Autodesk Fusion 360 part; units mm, degrees
sketch "Sketch1" plane through (0, 0, 0) normal (0, 0, 1) x (1, 0, 0)
  line L0 (-28, 37) -> (62, 37)
  line L1 (62, 37) -> (62, 18)
  line L2 (62, 18) -> (-28, 18)
  line L3 (-28, 18) -> (-28, 37)
  dimension "d1" = 90
  dimension "d2" = 19
extrude "Extrude1" add sketch "Sketch1" along normal blind 6
sketch "Sketch2" plane through (0, 0, 6) normal (0, 0, 1) x (-1, 0, 0)
  line L0 (28, -37) -> (28, -18)
  line L1 (28, -18) -> (-62, -18)
  line L2 (-62, -18) -> (-62, -37)
  line L3 (-62, -37) -> (28, -37)
ref_plane "WorkPlane1" through (17, 27.5, 6) normal (0, 0, 1) x (-1, 0, 0)
sketch "Sketch3" plane through (0, 0, 6) normal (0, 0, 1) x (1, 0, 0)
  line L0 (17, 37) -> (17, 18)
  circle A0 centre (-8, 27.5) radius 8.9
  circle A1 centre (42, 27.5) radius 8.9
  circle A2 centre (-8, 27.5) radius 3.65
  circle A3 centre (42, 27.5) radius 3.65
  dimension "d13" = 17.8
  dimension "d14" = 17.8
  dimension "d15" = 7.3
  dimension "d16" = 7.3
extrude "Extrude2" cut sketch "Sketch3" against normal blind 7 contours A2 | A3
extrude "Extrude3" cut sketch "Sketch3" against normal blind 3
sketch "Sketch4" plane through (0, 0, 0) normal (0, 0, 1) x (1, 0, 0)
  line L0 (-21, 37) -> (55, 37)
  line L1 (55, 37) -> (55, 39)
  line L2 (55, 39) -> (-21, 39)
  line L3 (-21, 39) -> (-21, 37)
  dimension "d21" = 76
  dimension "d22" = 2
sketch "Sketch7" plane through (0, 0, 6) normal (0, 0, 1) x (-1, 0, 0)
  circle A0 centre (-42, -27.5) radius 8.9
  circle A1 centre (8, -27.5) radius 8.9
  line L0 (28, -18) -> (-62, -18)
  line L1 (-62, -18) -> (-62, -37)
  line L2 (-62, -37) -> (28, -37)
  line L3 (28, -37) -> (28, -18)
  line L4 (28, -37) -> (-62, -37)
  line L5 (-62, -37) -> (-62, -73)
  line L6 (-62, -73) -> (28, -73)
  line L7 (28, -73) -> (28, -37)
  dimension "d37" = 90
  dimension "d38" = 36
extrude "Extrude7" add sketch "Sketch7" against normal blind 6 contours L2 L4 L5 L6 L7
sketch "Sketch8" plane through (0, 0, 6) normal (0, 0, 1) x (-1, 0, 0)
  circle A0 centre (-42, -27.5) radius 8.9
  circle A1 centre (8, -27.5) radius 8.9
  line L0 (28, -18) -> (-62, -18)
  line L1 (-62, -18) -> (-62, -73)
  line L2 (-62, -73) -> (28, -73)
  line L3 (28, -73) -> (28, -18)
  line L4 (-62, -18) -> (28, -18)
  line L5 (28, -18) -> (28, 18)
  line L6 (28, 18) -> (-62, 18)
  line L7 (-62, 18) -> (-62, -18)
  dimension "d41" = 90
  dimension "d42" = 36
extrude "Extrude8" add sketch "Sketch8" against normal blind 6 contours L0 L4 L5 L6 L7
ref_plane "WorkPlane3" through (17, 27.5, 6) normal (0, 0, 1) x (1, 0, 0)
sketch "Sketch9" plane through (0, 0, 6) normal (0, 0, 1) x (1, 0, 0)
  line L0 (62, -18) -> (-28, -18)
  line L1 (-28, -18) -> (-28, -14)
  line L2 (-28, -14) -> (62, -14)
  line L3 (62, -14) -> (62, -18)
  line L4 (62, 73) -> (-28, 73)
  line L5 (-28, 73) -> (-28, 69)
  line L6 (-28, 69) -> (62, 69)
  line L7 (62, 69) -> (62, 73)
  line L8 (62, -14) -> (62, -14)
  line L9 (62, 69) -> (62, 69)
  line L10 (62, -14) -> (58, -14)
  line L11 (58, -14) -> (58, 69)
  line L12 (58, 69) -> (62, 69)
  line L13 (62, 69) -> (62, -14)
  dimension "d46" = 90
  dimension "d47" = 4
  dimension "d48" = 90
  dimension "d49" = 4
  dimension "d50" = 83
extrude "Extrude9" add sketch "Sketch9" along normal blind 27
ref_plane "WorkPlane4" through (17, 27.5, 33) normal (0, 0, 1) x (1, 0, 0)
sketch "Sketch10" plane through (0, 0, 33) normal (0, 0, 1) x (1, 0, 0)
  line L0 (62, -18) -> (22, -18)
  line L1 (22, -18) -> (22, 73)
  line L2 (22, 73) -> (62, 73)
  line L3 (62, 73) -> (62, -18)
  line L4 (62, -18) -> (-28, -18)
  line L5 (-28, -18) -> (-28, 2)
  line L6 (-28, 2) -> (62, 2)
  line L7 (62, 2) -> (62, -18)
  line L8 (62, 73) -> (-28, 73)
  line L9 (-28, 73) -> (-28, 53)
  line L10 (-28, 53) -> (62, 53)
  line L11 (62, 53) -> (62, 73)
  dimension "d54" = 40
  dimension "d55" = 91
  dimension "d56" = 90
  dimension "d57" = 20
  dimension "d58" = 90
  dimension "d59" = 20
extrude "Extrude10" add sketch "Sketch10" along normal blind 4
fillet "Fillet3" radius 8 2 edges at (-28, 2, 35) (-28, 53, 35)
fillet "Fillet4" radius 8 1 edges at (22, 2, 35)
fillet "Fillet5" radius 8 1 edges at (22, 53, 35)
fillet "Fillet6" radius 2 2 edges at (62, -18, 18.5) (-28, -18, 18.5)
fillet "Fillet7" radius 2 7 edges at (-28, 73, 16.5) (-28, 73, 35) (-28, 73, 16.5) (-28, 73, 35) (62, 73, 16.5) (62, 73, 35) (62, 73, 16.5)
Design review of the part built by this model. Coordinates are the model's own, in mm. A direction names the side the tool comes from. Give positions to 0.01 mm unless a question says otherwise; leave off trailing zeros. Loops run counter-clockwise (first coordinate to the right, second up) from the corner with the lowest first, then second, coordinate; pieces in that order, holes last. Notation, with made-up numbers: (-8.75, 42) - (40.25, 42) arc R25 cw to (40.25, 66) - close; hole circle Ø10 at (-14, 2). An arc over 180 degrees is marked (long way). Use CSV: the item, a comma, the result in double quotes. Start each with the question number.
1. Add section D-D (x = 42). State the section outline as (y, z) points.
2. Draft analysis for pull direction X (two halves, no side actions). For faces 6 (the cylindrical face through (-25.594, -0.281, 35.028)), 7 (the cylindrical face through (39.103, 25.279, 1.521)), 8 (the flat face through (46, 28, 3)), 9 (the flat face through (24, 28, 33)), state which applies: released by +X, released by -X, zero draft, split by the parting line, or undercut.
3. Insertion check: P1, Ø5, axis at y = 56, z = 31, coming from the -X side; P2, Ø1.2, axis at y = 28.5, z = 35, coming from the -X side; P3, Ø1, axis at x = 12.5, y = 15.5, coming from the +Z side. Each pin has a flat end and moves straight along its axis. Give the tip position at first contact, or say it passes through.
4. Add section A-A (y = 27.5). State the section outline as (x, z) points, plus the area to 3 significant figures.
5. Machinability: for faces 1 (the flat face through (26, 28, 37)), 2 (the cylindrical face through (19.719, 50.594, 35.028)), 3 (the cylindrical face through (-3.9, 19.6, 4.5)), 4 (the cylindrical face through (61.43, -17.4, 18.24)), 5 (the flat face through (14, -14, 19)), which of the approach directions +Z, -Z, +X, -X, +Y, -Y give a long, thin tool a straight path to every point of the face, cutting with its end or side? Answer none if there is none.
6. Add section B-B (x = -8). State the section outline as (y, z) points.
7. Wall thickness on L1, parallel to Z at x = -21.5, y = 64; L2, parallel to Y at x = -8, z = 4.85; L3, parallel to X at y = 27, z = 4: over which ranges is each line inside the solid? List them lowest first.
8. Add section C-C (z = 25.5). State the section outline as (x, y) points.
Results found:
1,outline,"(-18, 0) - (23.85, 0) - (23.85, 3) - (18.6, 3) - (18.6, 6) - (-14, 6) - (-14, 33) - (69, 33) - (69, 6) - (36.4, 6) - (36.4, 3) - (31.15, 3) - (31.15, 0) - (73, 0) - (73, 37) - (-18, 37) - close"
2,face 6,"released by -X"
2,face 7,"undercut"
2,face 8,"undercut"
2,face 9,"zero draft"
3,P1,"stops at x = -27.19"
3,P2,"stops at x = 22"
3,P3,"stops at z = 6"
4,outline,"(-28, 0) - (-11.65, 0) - (-11.65, 3) - (-16.9, 3) - (-16.9, 6) - (-28, 6) - close; (-4.35, 0) - (38.35, 0) - (38.35, 3) - (33.1, 3) - (33.1, 6) - (0.9, 6) - (0.9, 3) - (-4.35, 3) - close; (22, 33) - (58, 33) - (58, 6) - (50.9, 6) - (50.9, 3) - (45.65, 3) - (45.65, 0) - (62, 0) - (62, 37) - (22, 37) - close"
4,area,"657 mm²"
5,face 1,"+Z, +X, -X, +Y, -Y"
5,face 2,"+Z, -X"
5,face 3,"+Z"
5,face 4,"+Z, -Z, +X, -Y"
5,face 5,"-X"
6,outline,"(-18, 0) - (23.85, 0) - (23.85, 3) - (18.6, 3) - (18.6, 6) - (-14, 6) - (-14, 33) - (2, 33) - (2, 37) - (-18, 37) - close; (31.15, 0) - (73, 0) - (73, 37) - (53, 37) - (53, 33) - (69, 33) - (69, 6) - (36.4, 6) - (36.4, 3) - (31.15, 3) - close"
7,L1,"z = 0 to 6, 33 to 37"
7,L2,"y = -18 to 18.6, 36.4 to 73"
7,L3,"x = -28 to -16.89, 0.89 to 33.11, 50.89 to 62"
8,outline,"(-28, -16) arc R2 ccw to (-26, -18) - (60, -18) arc R2 ccw to (62, -16) - (62, 71) arc R2 ccw to (60, 73) - (-26, 73) arc R2 ccw to (-28, 71) - (-28, 69) - (58, 69) - (58, -14) - (-28, -14) - close"
